Work out the finished part from the listing and answer in its coordinate system (mm). A direction names the side the tool comes from. Coordinates: 2 decimals unless noted, no trailing zeros. Write each loop counter-clockwise with the first axis right and the second up, starting at its lowest first coordinate (ties: lowest second). Pieces come first, ordered by that corner, then holes. Notation, with made-up numbers: (72, 0) - (117, 0) arc R32 ccw to (117, 29) - close; hole circle Ø8 at (67, 0.25). An arc over 180 degrees is marked (long way). Use a Markdown table: item, result. Add a question column.
(1) A tool of negligible diameter and unlimited length cuts with its end or side. For faces 1 (the face through (12.7, -1, 0)), 2 (the face through (-39, 0, 0)), 3 (the face through (0, -38, 0)), from which of +Z, -Z, +X, -X, +Y, -Y can it reach the whole face along a straight path? Write none if from no direction.
(2) Given pin 1 Ø2 at (x, z) = (-47.5, 0.5) entering from -Y; pin 2 Ø4 at (y, z) = (-37, 2.5) entering from -X, each flat-ended and moving along its own axis, determine where each tip first touches the part or whether it passes through.
(3) The part is cut by section C-C, the plane y = 37. Give the vertices of the cut face in (x, z).
(4) The part is cut by section A-A, the plane z = 2. Give the vertices of the cut face in (x, y), then the cut area to 3 significant figures.
(5) Find the intervals of material crossed by line 1 (X direction, y = -45.5, z = 4.25); line 2 (Y direction, x = -25, z = -2.25), in increasing order. Write a range as from..to.
(6) The part is cut by section B-B, the plane x = -49.5. Give the vertices of the cut face in (y, z).
from build123d import *

# Parameters (mm, degrees)
F0_W     = 127
F0_H     = 12.7
F1_DEPTH = 12.7
F2_W     = 76.2
F2_H     = 12.7
F3_DEPTH = 12.7


with BuildPart() as f1:
    # F0 (on Right) → F1 (new body)
    with BuildSketch(Plane.YZ):
        Rectangle(F0_W, F0_H)
    extrude(amount=F1_DEPTH)

    # F2 (on Front) → F3 (join)
    with BuildSketch(Plane.XZ):
        with Locations((-38.1, 0)):
            Rectangle(F2_W, F2_H)
    extrude(amount=F3_DEPTH)


solid = f1.part
Model answer:
| question | item | result |
|---|---|---|
| 1 | face 1 | +Z, -Z, +X, +Y, -Y |
| 1 | face 2 | +Z, -Z, -X, +Y |
| 1 | face 3 | +Z, -Z, -X, -Y |
| 2 | pin 1 | y = -12.7 |
| 2 | pin 2 | x = 0 |
| 3 | outline | (0, -6.35) - (12.7, -6.35) - (12.7, 6.35) - (0, 6.35) - close |
| 4 | outline | (-76.2, -12.7) - (0, -12.7) - (0, -63.5) - (12.7, -63.5) - (12.7, 63.5) - (0, 63.5) - (0, 0) - (-76.2, 0) - close |
| 4 | area | 2,580 mm^2 |
| 5 | line 1 | 0..12.7 |
| 5 | line 2 | -12.7..0 |
| 6 | outline | (-12.7, -6.35) - (0, -6.35) - (0, 6.35) - (-12.7, 6.35) - close |
